Source: CAD feature listing. Evaluate the final solid. Frame: model axes, mm. A direction names the side the tool comes from. Give positions to 0.01 mm unless a question says otherwise; leave off trailing zeros. Loops run counter-clockwise (first coordinate to the right, second up) from the corner with the lowest first, then second, coordinate; pieces in that order, holes last. Notation, with made-up numbers: M -6.75,-22 L 37.25,-22 A33 cw 37.25,9 Z; hole C 87.5,12.25 d2. An arc over 180 degrees is marked long. Put each result on its own line as item: value.
from build123d import *

# Parameters (mm, degrees)
SKETCH1_R           = 2
BOSS_EXTRUDE1_DEPTH = 5
CUT_EXTRUDE1_DEPTH  = 2


with BuildPart() as part:
    # Sketch1 → Boss-Extrude1 (new body)
    with BuildSketch(Plane(origin=(0, 0, 0), x_dir=(1, 0, 0), z_dir=(0, 1, 0))):
        with BuildLine():
            Line((-68.767020688, 12.176966292), (63.205222935, 12.176966292))
            ThreePointArc((63.205222935, 12.176966292), (65.877835354, 12.540725176), (68.356010471, 13.605537721))
            ThreePointArc((68.356010471, 13.605537721), (79.719101124, 7.176966292), (68.356010471, 0.748394864))
            ThreePointArc((68.356010471, 0.748394864), (65.877835354, 1.813207409), (63.205222935, 2.176966292))
            Line((63.205222935, 2.176966292), (-68.767020688, 2.176966292))
            ThreePointArc((-68.767020688, 2.176966292), (-71.439633107, 1.813207409), (-73.917808224, 0.748394864))
            ThreePointArc((-73.917808224, 0.748394864), (-85.280898876, 7.176966292), (-73.917808224, 13.605537721))
            ThreePointArc((-73.917808224, 13.605537721), (-71.439633107, 12.540725176), (-68.767020688, 12.176966292))
        make_face()
        with Locations(Location((-77.780898876, 7.176966292, 0), (0, 0, 270))):
            Circle(SKETCH1_R, mode=Mode.SUBTRACT)
        with Locations(Location((72.219101124, 7.176966292, 0), (0, 0, 270))):
            Circle(SKETCH1_R, mode=Mode.SUBTRACT)
    extrude(amount=BOSS_EXTRUDE1_DEPTH)

    # Sketch3 → Cut-Extrude1 (cut)
    with BuildSketch(Plane(origin=(0, 5, 0), x_dir=(1, 0, 0), z_dir=(0, 1, 0))):
        with BuildLine():
            Line((-64.780898876, 9.676966292), (59.219101124, 9.676966292))
            ThreePointArc((59.219101124, 9.676966292), (61.719101124, 7.176966292), (59.219101124, 4.676966292))
            Line((59.219101124, 4.676966292), (-64.780898876, 4.676966292))
            ThreePointArc((-64.780898876, 4.676966292), (-67.280898876, 7.176966292), (-64.780898876, 9.676966292))
        make_face()
    extrude(amount=-CUT_EXTRUDE1_DEPTH, mode=Mode.SUBTRACT)


solid = part.part
1. Contact query for flat-ended pins moving along their axis: P1, Ø4, axis at x = -25, z = -7.5, coming from the +Y side; P2, Ø3.5, axis at x = -77.78, z = -7.18, coming from the -Y side; P3, Ø1.6, axis at x = 4.5, y = 4.5, coming from the +Z side; P4, Ø1.6, axis at x = 27.5, y = 4, coming from the -Z side. Output: stop coordinate, or through.
Found:
P1: y = 3
P2: through
P3: z = -2.18
P4: z = -12.18
2. Access query for faces 4 (the cylindrical face through (65.84, 2.46, -12.53)), 5 (the cylindrical face through (-71.403, 2.465, -1.823)), 6 (the cylindrical face through (61.72, 4.01, -7.23)), 7 (the cylindrical face through (70.267, 2.465, -7.611)). Directions: +Z, -Z, +X, -X, +Y, -Y. A direction counts if a zero-diameter tool reaches every point of the face in a straight line with its end or side. Return the directions, or none.
Found:
face 4: -Z, +Y, -Y
face 5: +Z, +Y, -Y
face 6: +Y
face 7: +Y, -Y
3. Section query B-B (x = -4). Output: boundary loops of the cut face in (y, z), plus the area to 3 significant figures.
Found:
outline: M 0,-12.18 L 5,-12.18 L 5,-9.68 L 3,-9.68 L 3,-4.68 L 5,-4.68 L 5,-2.18 L 0,-2.18 Z
area: 40.0 mm^2
4. Draft query along Z for faces 1 (the flat face through (-2, 5, -4)), 2 (the flat face through (-4, 2, -12.177)), 3 (the flat face through (-2, 3, -7)). Return one class per face: pulls with the +Z half, pulls with the -Z half, needs draft (parallel to the pull), parting line crosses it, or undercut.
Found:
face 1: needs draft
face 2: pulls with the -Z half
face 3: undercut
5. Material intervals for line 1 (X direction, y = 1.95, z = -7.25); line 2 (X direction, y = 3.8, z = -9); line 3 (X direction, y = 2.2, z = -6.5), sorted ascending. Write a range as from..to.
Found:
line 1: -85.28..-79.78, -75.78..70.22, 74.22..79.72
line 2: -85.06..-78.6, -76.96..-66.49, 60.93..71.4, 73.04..79.49
line 3: -85.25..-79.66, -75.9..70.34, 74.1..79.69
6. Section query A-A (y = 4.05). Output: boundary loops of the cut face in (x, z), plus the area to 3 significant figures.
Found:
outline: M -73.92,-13.61 A10 cw -68.77,-12.18 L 63.21,-12.18 A10 cw 68.36,-13.61 A7.5 ccw long 68.36,-0.75 A10 cw 63.21,-2.18 L -68.77,-2.18 A10 cw -73.92,-0.75 A7.5 ccw long Z; hole C -77.78,-7.18 d4; hole M -64.78,-9.68 L 59.22,-9.68 A2.5 ccw 59.22,-4.68 L -64.78,-4.68 A2.5 ccw Z; hole C 72.22,-7.18 d4
area: 1,050 mm^2
